Check sheet for the modelled part. Datum: model origin and axes. Units: mm. Give positions to 0.01 mm unless a question says otherwise; leave off trailing zeros. Loops run counter-clockwise (first coordinate to the right, second up) from the corner with the lowest first, then second, coordinate; pieces in that order, holes last. Notation, with made-up numbers: (82, 32) -> (93, 32) arc R27 cw to (93, 57) -> close; hole circle Ø3 at (57, 55). An arc over 180 degrees is marked (long way). Write each question's results on one line, items separated by ' | '. Start each with the question number.
1. Cross-section at B-B on z = 3.7. Count the separate pieces of the cut face and the enclosed holes in it, and give its area (3 significant figures).
2. Cross-section at C-C on y = -133.5. Record the boundary of the cut face in (x, z).
3. Gauge pin test, flat ends, axial feed: pin 1 Ø2.5 at (x, y) = (-5.5, -140) entering from +Z; pin 2 Ø1.5 at (x, z) = (-96.5, 2) entering from -Y; pin 3 Ø1.5 at (x, z) = (-150.5, 3) entering from -Y; pin 4 Ø2.5 at (x, z) = (-307, 2.5) entering from -Y. Record the tip position at first contact, or that the pin passes through.
4. Material ranges on L1, parallel to Y at x = -15.5, z = 2.85; L2, parallel to Y at x = -25.5, z = 1.9; L3, parallel to Y at x = -27, z = 2.7, recorded low to high. Write a range as from..to.
5. Cross-section at A-A on y = -32.5. Record the boundary of the cut face in (x, z), and give its area (3 significant figures).
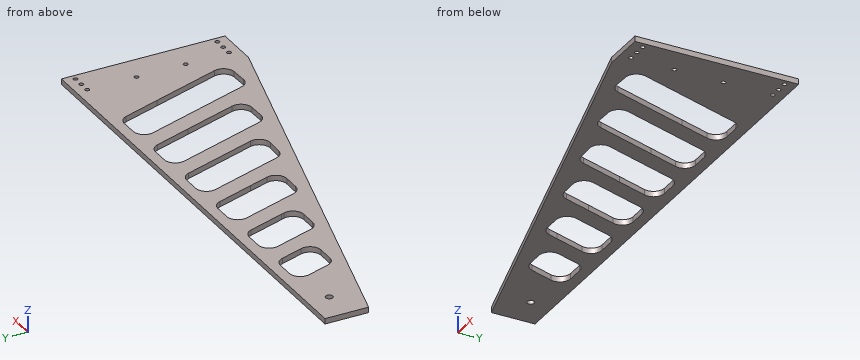
from build123d import *

# Parameters (mm, degrees)
AUFSATZ_LINEAR_AUSTRAGEN1_DEPTH  = 5
SKIZZE2_R                        = 3.25
SCHNITT_LINEAR_AUSTRAGEN1_DEPTH  = 6
F_4_0_4_DURCHMESSER_BOHRUNG1_D   = 4
F_4_1_4_1_DURCHMESSER_BOHRUNG1_D = 4.1
SCHNITT_LINEAR_AUSTRAGEN2_DEPTH  = 8


with BuildPart() as part:
    # Skizze1 → Aufsatz-Linear austragen1 (new body)
    with BuildSketch(Plane.XY):
        Polygon((0, 0), (0, -150), (-40, -150), (-450, -40), (-450, 0), align=None)
    extrude(amount=AUFSATZ_LINEAR_AUSTRAGEN1_DEPTH)

    # Skizze2 → Schnitt-Linear austragen1 (cut, through all)
    with BuildSketch(Plane.XY.offset(5)):
        with Locations((-420, -20)):
            Circle(SKIZZE2_R)
    extrude(amount=-SCHNITT_LINEAR_AUSTRAGEN1_DEPTH, mode=Mode.SUBTRACT)

    # Ø4.0 (4) Durchmesser Bohrung1 (through all)
    with Locations(Plane.XY.offset(5)):
        with Locations((-25.5, -10), (-15.5, -10), (-5.5, -10), (-5.5, -140), (-15.5, -140), (-25.5, -140)):
            Hole(F_4_0_4_DURCHMESSER_BOHRUNG1_D / 2)

    # Ø4.1 (4.1) Durchmesser Bohrung1 (through all)
    with Locations(Plane(origin=(0, 0, 0), x_dir=(-1, 0, 0), z_dir=(0, 0, -1))):
        with Locations((26, -55), (26, -100)):
            Hole(F_4_1_4_1_DURCHMESSER_BOHRUNG1_D / 2)

    # Skizze9 → Schnitt-Linear austragen2 (cut)
    with BuildSketch(Plane.XY.offset(5)):
        with BuildLine():
            Line((-103.931576355, -10), (-88.847327603, -10))
            ThreePointArc((-88.847327603, -10), (-83.003068108, -11.885529533), (-79.362713389, -16.831073809))
            Line((-79.362713389, -16.831073809), (-67.965211215, -50.943863007))
            Line((-67.965211215, -50.943863007), (-46.397909384, -115.49492075))
            ThreePointArc((-46.397909384, -115.49492075), (-47.662174175, -124.358217438), (-55.515574608, -128.657112095))
            Line((-55.515574608, -128.657112095), (-70.41700546, -129.20428711))
            ThreePointArc((-70.41700546, -129.20428711), (-76.478324948, -127.43137138), (-80.268568666, -122.379948147))
            Line((-80.268568666, -122.379948147), (-104.136242779, -50.943863007))
            Line((-104.136242779, -50.943863007), (-113.416190569, -23.168926191))
            ThreePointArc((-113.416190569, -23.168926191), (-112.046046821, -14.155740505), (-103.931576355, -10))
        make_face()
        with BuildLine():
            Line((-132.659135945, -16.831073809), (-121.261633772, -50.943863007))
            Line((-121.261633772, -50.943863007), (-104.819891238, -100.154092454))
            ThreePointArc((-104.819891238, -100.154092454), (-106.1314685, -109.085090058), (-114.102677631, -113.320981714))
            Line((-114.102677631, -113.320981714), (-129.085869406, -113.62344582))
            ThreePointArc((-129.085869406, -113.62344582), (-135.049768642, -111.798519703), (-138.772311443, -106.794408942))
            Line((-138.772311443, -106.794408942), (-157.432665335, -50.943863007))
            Line((-157.432665335, -50.943863007), (-166.712613125, -23.168926191))
            ThreePointArc((-166.712613125, -23.168926191), (-165.342469378, -14.155740505), (-157.227998911, -10))
            Line((-157.227998911, -10), (-142.14375016, -10))
            ThreePointArc((-142.14375016, -10), (-136.299490665, -11.885529533), (-132.659135945, -16.831073809))
        make_face()
        with BuildLine():
            Line((-185.955558502, -16.831073809), (-174.558056328, -50.943863007))
            Line((-174.558056328, -50.943863007), (-162.967615916, -85.634117455))
            ThreePointArc((-162.967615916, -85.634117455), (-164.435252335, -94.780339607), (-172.782043853, -98.797603311))
            Line((-172.782043853, -98.797603311), (-188.034457791, -98.294283947))
            ThreePointArc((-188.034457791, -98.294283947), (-193.68194003, -96.316702077), (-197.189258283, -91.468650472))
            Line((-197.189258283, -91.468650472), (-210.729087892, -50.943863007))
            Line((-210.729087892, -50.943863007), (-220.009035682, -23.168926191))
            ThreePointArc((-220.009035682, -23.168926191), (-218.638891934, -14.155740505), (-210.524421467, -10))
            Line((-210.524421467, -10), (-195.440172716, -10))
            ThreePointArc((-195.440172716, -10), (-189.595913221, -11.885529533), (-185.955558502, -16.831073809))
        make_face()
        with BuildLine():
            Line((-239.251981058, -16.831073809), (-227.854478884, -50.943863007))
            Line((-227.854478884, -50.943863007), (-221.703520719, -69.353715979))
            ThreePointArc((-221.703520719, -69.353715979), (-223.095303096, -78.396829164), (-231.261995944, -82.522369394))
            Line((-231.261995944, -82.522369394), (-246.383562521, -82.410676928))
            ThreePointArc((-246.383562521, -82.410676928), (-252.183888505, -80.503781541), (-255.794315725, -75.579875894))
            Line((-255.794315725, -75.579875894), (-264.025510448, -50.943863007))
            Line((-264.025510448, -50.943863007), (-273.305458238, -23.168926191))
            ThreePointArc((-273.305458238, -23.168926191), (-271.93531449, -14.155740505), (-263.820844024, -10))
            Line((-263.820844024, -10), (-248.736595273, -10))
            ThreePointArc((-248.736595273, -10), (-242.892335777, -11.885529533), (-239.251981058, -16.831073809))
        make_face()
        with BuildLine():
            Line((-292.548403615, -16.831073809), (-281.150901441, -50.943863007))
            Line((-281.150901441, -50.943863007), (-280.31760719, -53.437917466))
            ThreePointArc((-280.31760719, -53.437917466), (-281.68198, -62.443082132), (-289.782458776, -66.606824129))
            Line((-289.782458776, -66.606824129), (-304.856754045, -66.636614958))
            ThreePointArc((-304.856754045, -66.636614958), (-310.712755148, -64.75687589), (-314.361130888, -59.805560676))
            Line((-314.361130888, -59.805560676), (-317.321933004, -50.943863007))
            Line((-317.321933004, -50.943863007), (-326.601880795, -23.168926191))
            ThreePointArc((-326.601880795, -23.168926191), (-325.231737047, -14.155740505), (-317.11726658, -10))
            Line((-317.11726658, -10), (-302.033017829, -10))
            ThreePointArc((-302.033017829, -10), (-296.188758334, -11.885529533), (-292.548403615, -16.831073809))
        make_face()
        with BuildLine():
            Line((-345.844826171, -16.831073809), (-338.847224106, -37.774936817))
            ThreePointArc((-338.847224106, -37.774936817), (-340.217367853, -46.788122502), (-348.33183832, -50.943863007))
            Line((-348.33183832, -50.943863007), (-363.416087071, -50.943863007))
            ThreePointArc((-363.416087071, -50.943863007), (-369.260346566, -49.058333474), (-372.900701286, -44.112789198))
            Line((-372.900701286, -44.112789198), (-379.898303351, -23.168926191))
            ThreePointArc((-379.898303351, -23.168926191), (-378.528159603, -14.155740505), (-370.413689137, -10))
            Line((-370.413689137, -10), (-355.329440386, -10))
            ThreePointArc((-355.329440386, -10), (-349.48518089, -11.885529533), (-345.844826171, -16.831073809))
        make_face()
    extrude(amount=-SCHNITT_LINEAR_AUSTRAGEN2_DEPTH, mode=Mode.SUBTRACT)


solid = part.part
Geometry says:
1) separate pieces: 1 | enclosed holes: 15 | area: 28,100 mm^2
2) outline: (-101.5, 0) -> (0, 0) -> (0, 5) -> (-101.5, 5) -> close
3) pin 1: through | pin 2: y = -135.04 | pin 3: y = -120.55 | pin 4: y = -78.7
4) L1: -150..-142, -138..-12, -8..0 | L2: -150..-142, -138..-101.99, -98.01..-56.99, -53.01..-12, -8..0 | L3: -150..-141.32, -138.68..-101.79, -98.21..-56.79, -53.21..-11.32, -8.68..0
5) outline: (-450, 0) -> (-376.78, 0) -> (-376.78, 5) -> (-450, 5) -> close; (-340.61, 0) -> (-323.48, 0) -> (-323.48, 5) -> (-340.61, 5) -> close; (-287.31, 0) -> (-270.19, 0) -> (-270.19, 5) -> (-287.31, 5) -> close; (-234.02, 0) -> (-216.89, 0) -> (-216.89, 5) -> (-234.02, 5) -> close; (-180.72, 0) -> (-163.59, 0) -> (-163.59, 5) -> (-180.72, 5) -> close; (-127.42, 0) -> (-110.3, 0) -> (-110.3, 5) -> (-127.42, 5) -> close; (-74.13, 0) -> (0, 0) -> (0, 5) -> (-74.13, 5) -> close | area: 1,160 mm^2
